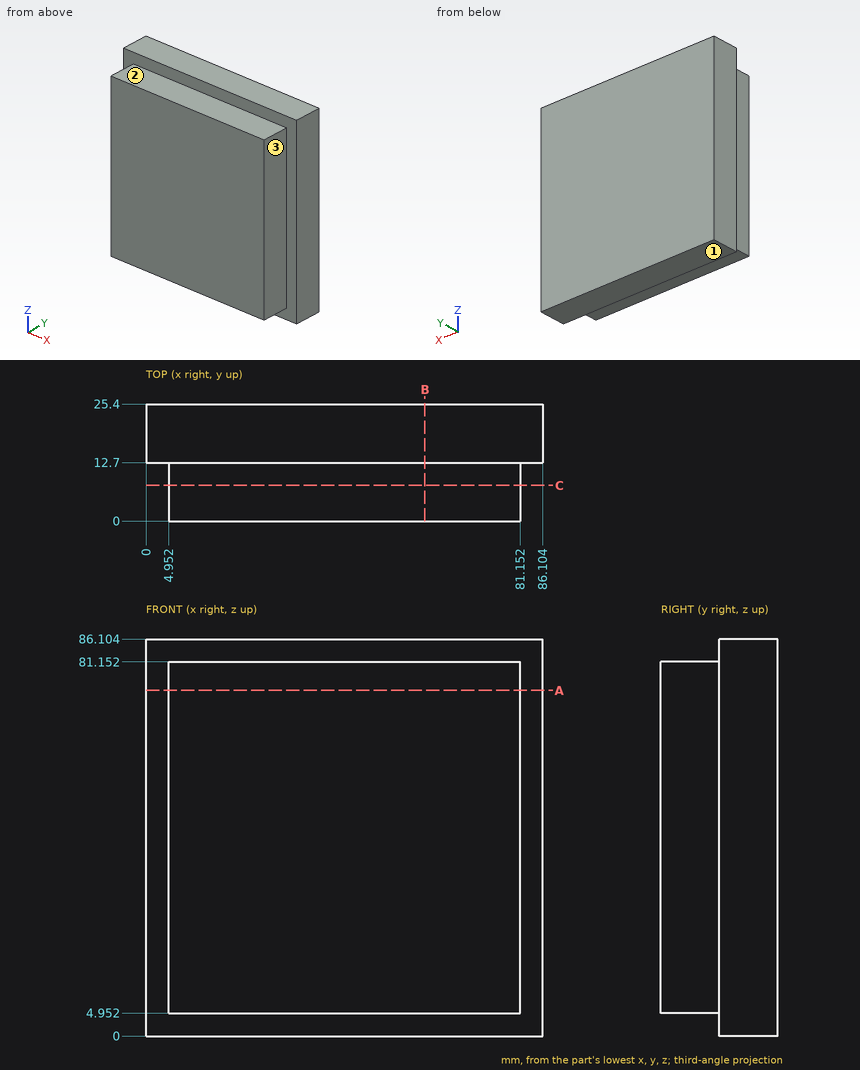
Geometry: see drawing. Coordinates: mm, zero at the bounding-box minimum. A direction names the side the tool comes from. Round coordinates to 2 decimals unless told otherwise and drop trailing zeros. Loops run counter-clockwise (first coordinate to the right, second up) from the corner with the lowest first, then second, coordinate; pieces in that order, holes last. Notation, with made-up numbers: (0, 73.5) - (20, 73.5) arc R22 cw to (20, 105.5) - close; hole circle Ø5 at (85, 21). An arc over 180 degrees is marked (long way). One line per item, written item: value. Start each with the question number.
(1) Section C-C, the plane y = 7.75. Return loops of the section in (x, z), plus the area to 3 significant figures.
(2) Ray query, line 1 (Z direction, x = 7, y = 4.5). Return the intervals inside material, ascending. Write a range as [from, to].
(3) Section B-B, the plane x = 60.5. Return loops of the section in (y, z), plus the area to 3 significant figures.
(4) Access query for the marked faces 1, 2 and 3. Directions: +Z, -Z, +X, -X, +Y, -Y. A direction counts if a zero-diameter tool reaches every point of the face in a straight line with its end or side. Return the directions, or none.
(5) Section A-A, the plane z = 75. Return loops of the section in (x, y).
(6) Contact query for flat-ended pins moving along their axis: P1, Ø6.5, axis at x = 32.5, y = 9, coming from the -Z side; P2, Ø3, axis at x = 21.5, y = 7, coming from the +Z side; P3, Ø14, axis at y = 4.5, z = 52.5, coming from the -X side. Output: stop coordinate, or through.
Results below:
1. outline: (4.95, 4.95) - (81.15, 4.95) - (81.15, 81.15) - (4.95, 81.15) - close
1. area: 5,810 mm^2
2. line 1: [4.95, 81.15]
3. outline: (0, 4.95) - (12.7, 4.95) - (12.7, 0) - (25.4, 0) - (25.4, 86.1) - (12.7, 86.1) - (12.7, 81.15) - (0, 81.15) - close
3. area: 2,060 mm^2
4. face 1: -Z, +X, -X, +Y, -Y
4. face 2: +Z, +X, -X, -Y
4. face 3: +Z, -Z, +X, -Y
5. outline: (0, 12.7) - (4.95, 12.7) - (4.95, 0) - (81.15, 0) - (81.15, 12.7) - (86.1, 12.7) - (86.1, 25.4) - (0, 25.4) - close
6. P1: z = 4.95
6. P2: z = 81.15
6. P3: x = 4.95
